Design review of the part built by this model. Coordinates are the model's own, in mm. A direction names the side the tool comes from. Coordinates: 2 decimals unless noted, no trailing zeros. Write each loop counter-clockwise with the first axis right and the second up, starting at its lowest first coordinate (ties: lowest second). Pieces come first, ordered by that corner, then holes. Notation, with made-up numbers: M 10.5,34.25 L 25.5,34.25 A14 cw 25.5,42.25 Z; hole C 76,46 d4. An arc over 180 degrees is marked long. Write each question's results on one line, items separated by ' | '. Start each with the question number.
```python
from build123d import *

# Parameters (mm, degrees)
BOX002_W          = 2.54
BOX002_H          = 12.7
BOX002_DEPTH      = 2.54
CYLINDER_R        = 0.35
CYLINDER_DEPTH    = 17
CYLINDER001_R     = 0.35
CYLINDER001_DEPTH = 17
CYLINDER002_R     = 0.35
CYLINDER002_DEPTH = 17
CYLINDER003_R     = 0.35
CYLINDER003_DEPTH = 17
CYLINDER004_R     = 0.35
CYLINDER004_DEPTH = 17
BOX001_W          = 20
BOX001_H          = 20
BOX001_DEPTH      = 6
FILLET_R          = 1
BOX003_W          = 2.54
BOX003_H          = 12.7
BOX003_DEPTH      = 6
PAD_DEPTH         = 1
SKETCH002_W       = 20.378432
SKETCH002_H       = 20.250089
PAD001_DEPTH      = 0.5
PAD002_DEPTH      = 1
BOX_W             = 25.4
BOX_H             = 25.4
BOX_DEPTH         = 0.7


with BuildPart() as obj1:
    # Box002 → Box002 (new body)
    with BuildSketch(Plane(origin=(0, 6.35, -2.5), x_dir=(1, 0, 0), z_dir=(0, 0, 1))):
        with Locations((1.27, 6.35)):
            Rectangle(BOX002_W, BOX002_H)
    extrude(amount=BOX002_DEPTH)


with BuildPart() as zylinder:
    # Cylinder → Cylinder (new body)
    with BuildSketch(Plane(origin=(1.27, 10.1, -16), x_dir=(1, 0, 0), z_dir=(0, 0, 1))):
        Circle(CYLINDER_R)
    extrude(amount=CYLINDER_DEPTH)


with BuildPart() as zylinder001:
    # Cylinder001 → Cylinder001 (new body)
    with BuildSketch(Plane(origin=(1.27, 12.64, -16), x_dir=(1, 0, 0), z_dir=(0, 0, 1))):
        Circle(CYLINDER001_R)
    extrude(amount=CYLINDER001_DEPTH)


with BuildPart() as zylinder002:
    # Cylinder002 → Cylinder002 (new body)
    with BuildSketch(Plane(origin=(1.27, 7.56, -16), x_dir=(1, 0, 0), z_dir=(0, 0, 1))):
        Circle(CYLINDER002_R)
    extrude(amount=CYLINDER002_DEPTH)


with BuildPart() as zylinder003:
    # Cylinder003 → Cylinder003 (new body)
    with BuildSketch(Plane(origin=(1.27, 15.18, -16), x_dir=(1, 0, 0), z_dir=(0, 0, 1))):
        Circle(CYLINDER003_R)
    extrude(amount=CYLINDER003_DEPTH)


with BuildPart() as zylinder004:
    # Cylinder004 → Cylinder004 (new body)
    with BuildSketch(Plane(origin=(1.27, 17.72, -16), x_dir=(1, 0, 0), z_dir=(0, 0, 1))):
        Circle(CYLINDER004_R)
    extrude(amount=CYLINDER004_DEPTH)


with BuildPart() as fillet_body:
    # Box001 → Box001 (new body)
    with BuildSketch(Plane(origin=(2.64, 2.7, -6), x_dir=(1, 0, 0), z_dir=(0, 0, 1))):
        with Locations((10, 10)):
            Rectangle(BOX001_W, BOX001_H)
    extrude(amount=BOX001_DEPTH)

    # Fillet
    fillet_edges = [fillet_body.edges().sort_by_distance(p)[0] for p in [
        (2.64, 12.7, -6),
        (22.64, 12.7, -6),
        (12.64, 2.7, -6),
        (12.64, 22.7, -6),
    ]]
    fillet(fillet_edges, radius=FILLET_R)


with BuildPart() as obj2:
    # Box003 → Box003 (new body)
    with BuildSketch(Plane(origin=(0, 6.35, -12.66), x_dir=(1, 0, 0), z_dir=(0, 0, 1))):
        with Locations((1.27, 6.35)):
            Rectangle(BOX003_W, BOX003_H)
    extrude(amount=BOX003_DEPTH)


with BuildPart() as body:
    # Sketch001 → Pad (new body)
    with BuildSketch(Plane.XY):
        Polygon((-18.85, 18.85), (-16.25, 18.85), (-16.25, 17.55), (-13.65, 17.55), (-13.65, 20.8), (-11.7, 20.8), (-11.7, 17.55), (-9.1, 17.55), (-9.1, 18.85), (-6.5, 18.85), (-6.5, 15.6), (-9.1, 15.6), (-9.1, 16.9), (-11.7, 16.9), (-11.7, 13.65), (-13.65, 13.65), (-13.65, 16.9), (-16.25, 16.9), (-16.25, 15.6), (-18.85, 15.6), align=None)
    extrude(amount=PAD_DEPTH)


with BuildPart() as body_1:
    # Body placement: moved
    add(body.part.moved(Location((25.4, 0, 0))))


with BuildPart() as body001:
    # Sketch002 → Pad001 (new body)
    with BuildSketch(Plane.XY):
        with Locations((-12.729216, 12.665044)):
            Rectangle(SKETCH002_W, SKETCH002_H)
    extrude(amount=PAD001_DEPTH)


with BuildPart() as body001_1:
    # Body001 placement: moved
    add(body001.part.moved(Location((25.5, 0, 0.4))))


with BuildPart() as body002:
    # Sketch003 → Pad002 (new body)
    with BuildSketch(Plane.XY):
        Polygon((-18.85, 18.85), (-16.25, 18.85), (-16.25, 17.55), (-13.65, 17.55), (-13.65, 20.8), (-11.7, 20.8), (-11.7, 17.55), (-9.1, 17.55), (-9.1, 18.85), (-6.5, 18.85), (-6.5, 15.6), (-9.1, 15.6), (-9.1, 16.9), (-11.7, 16.9), (-11.7, 13.65), (-13.65, 13.65), (-13.65, 16.9), (-16.25, 16.9), (-16.25, 15.6), (-18.85, 15.6), align=None)
    extrude(amount=PAD002_DEPTH)


with BuildPart() as body002_1:
    # Body002 placement: moved
    add(body002.part.moved(Location((25.5, -8.1, 0))))


with BuildPart() as fusion:
    # Box → Box (new body)
    with BuildSketch(Plane.XY):
        with Locations((12.7, 12.7)):
            Rectangle(BOX_W, BOX_H)
    extrude(amount=BOX_DEPTH)

    # Fusion: union obj1, Zylinder, Zylinder001, Zylinder002, Zylinder003, Zylinder004, Fillet body, obj2, Body, Body001, Body002
    add(obj1.part)
    add(zylinder.part)
    add(zylinder001.part)
    add(zylinder002.part)
    add(zylinder003.part)
    add(zylinder004.part)
    add(fillet_body.part)
    add(obj2.part)
    add(body_1.part)
    add(body001_1.part)
    add(body002_1.part)


solid = fusion.part
```
Item 1: Insertion check: pin 1 Ø6 at (x, y) = (7.5, 3.5) entering from -Z; pin 2 Ø6 at (x, z) = (16, -4.5) entering from -Y; pin 3 Ø1.5 at (x, z) = (4, -4) entering from +Y. Each pin has a flat end and moves straight along its axis. Give the tip position at first contact, or say it passes through.
Item 2: We need section C-C on x = 1.27. Count the separate pieces of the cut face and the enclosed holes in it, then the cut area to 3 significant figures.
Item 3: Draft analysis for pull direction X (two halves, no side actions). For faces 6 (the cylindrical face through (2.925, 12.84, -5.699)), 7 (the flat face through (0, 13, -1)), 8 (the flat face through (2, 13, -12.66)), state which applies: released by +X, released by -X, zero draft, split by the parting line, or undercut.
Item 4: We need section B-B on x = 12.75. State the section outline as (y, z) points, then the cut area to 3 significant figures.
Item 5: We need section D-D on z = -10.25. State the section outline as (x, y) points.
Item 6: For faces 1 (the flat face through (2.64, 13, -3)), 2 (the flat face through (1, 19.05, -1)), 3 (the flat face through (13, 2.7, -3)), 4 (the flat face through (22.64, 13, -3)), 5 (the flat face through (1, 6.35, -1)), list the 3-axis set-ups (+Z, -Z, +X, -X, +Y, -Y) from which the entire face can be reached by the end or side of a thin tool; tool diameter is ignored.
Item 7: We need section A-A on y = 5. State the section outline as (x, z) points, then the cut area to 3 significant figures.
Item 8: Wall thickness on L1, parallel to Z at x = 1.5, y = 16; L2, parallel to Y at x = 9.75, z = -0.75; L3, parallel to Z at x = 10.75, y = 7.5: over which ranges is each line inside the solid? List them lowest first.
Answer:
1) pin 1: stops at z = -6 | pin 2: stops at y = 2.7 | pin 3: stops at y = 22.7
2) separate pieces: 1 | enclosed holes: 4 | area: 153 mm^2
3) face 6: undercut | face 7: released by -X | face 8: zero draft
4) outline: M 0,0 L 2.7,0 L 2.7,-5 A1 ccw 3.7,-6 L 21.7,-6 A1 ccw 22.7,-5 L 22.7,0 L 25.4,0 L 25.4,0.7 L 22.79,0.7 L 22.79,0.9 L 20.8,0.9 L 20.8,1 L 13.65,1 L 13.65,0.9 L 12.7,0.9 L 12.7,1 L 5.55,1 L 5.55,0.9 L 2.54,0.9 L 2.54,0.7 L 0,0.7 Z | area: 143 mm^2
5) outline: M 0,6.35 L 2.54,6.35 L 2.54,19.05 L 0,19.05 Z
6) face 1: -Z, +Y, -Y | face 2: -Z, -X, +Y | face 3: -Z, +X, -X, -Y | face 4: -Z, +X, +Y, -Y | face 5: -Z, -X, -Y
7) outline: M 0,0 L 2.64,0 L 2.64,-5 A1 ccw 3.64,-6 L 21.64,-6 A1 ccw 22.64,-5 L 22.64,0 L 25.4,0 L 25.4,0.7 L 22.96,0.7 L 22.96,0.9 L 2.58,0.9 L 2.58,0.7 L 0,0.7 Z | area: 141 mm^2
8) L1: z = -12.66 to -6.66, -2.5 to 0.7 | L2: y = 2.7 to 22.7 | L3: z = -6 to 0.9
